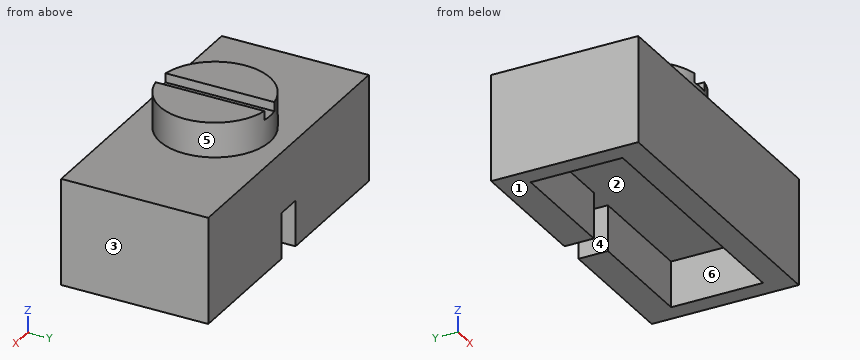
```python
from build123d import *

# Parameters (mm, degrees)
PAD_DEPTH    = 2.5
SKETCH001_W  = 16
SKETCH001_H  = 8
PAD001_DEPTH = 3.3
SKETCH002_R  = 3
PAD002_DEPTH = 5.2
SKETCH003_W  = 1
SKETCH003_H  = 8
POCKET_DEPTH = 0.5


with BuildPart() as part:
    # Sketch → Pad (new body)
    with BuildSketch(Plane.XY):
        Polygon((-8, 4), (-8, -4), (8, -4), (8, 4), (0.7, 4), (0.7, 2.4), (7, 2.4), (7, -2.6), (-7, -2.6), (-7, 2.4), (-0.7, 2.4), (-0.7, 4), align=None)
    extrude(amount=-PAD_DEPTH)

    # Sketch001 → Pad001 (join)
    with BuildSketch(Plane.XY):
        Rectangle(SKETCH001_W, SKETCH001_H)
    extrude(amount=PAD001_DEPTH)

    # Sketch002 → Pad002 (join)
    with BuildSketch(Plane.XY):
        Circle(SKETCH002_R)
    extrude(amount=PAD002_DEPTH)

    # Sketch003 (on Face10 of Pad002) → Pocket (cut)
    with BuildSketch(Plane.XY.offset(5.2)):
        Rectangle(SKETCH003_W, SKETCH003_H)
    extrude(amount=-POCKET_DEPTH, mode=Mode.SUBTRACT)


solid = part.part
```
CAD build for the part. Positions are in the model's coordinates, mm. Face numbers are marked on the shaded views. A direction names the side the tool comes from. Give positions to 0.01 mm unless a question says otherwise; leave off trailing zeros. Write each loop counter-clockwise with the first axis right and the second up, starting at its lowest first coordinate (ties: lowest second). Pieces come first, ordered by that corner, then holes. Notation, with made-up numbers: M 42,6.5 L 65,6.5 A30 cw 65,35.5 Z; hole C 13,-39 d5. An arc over 180 degrees is marked long. Return JSON: item names as keys, results as strings. Group by question number.
(1) Band-saw the part on D-D (x = 5). Give the cut face in (y, z).
(2) 3-axis set-ups, long thin cutter, end or side, ignore diameter. For the marked faces 4, 5 and 6: which of +Z, -Z, +X, -X, +Y, -Y reach the whole face in a straight line?
(3) Band-saw the part on C-C (z = -1). Give the cut face in (x, y).
(4) Flat gauge pins, fed straight in: pin 1 Ø2 at (x, y) = (-5.5, -3) entering from +Z; pin 2 Ø2 at (x, y) = (-0.5, 0.5) entering from -Z; pin 3 Ø0.5 at (x, y) = (0, 0.5) entering from +Z. Where does each tip first touch, or does it go through?
(5) Mould opens along X. For the marked faces 1, 2 and 3 say: pulls with the +X half, pulls with the -X half, needs draft (parallel to the pull), parting line crosses it, or undercut.
(6) Band-saw the part on A-A (x = 0). Give the cut face in (y, z).
(7) Band-saw the part on B-B (y = 0). Give the cut face in (x, z), and give its area (3 significant figures).
(8) Drill centre lines: L1, parallel to Y at x = 3.5, z = -0.25; L2, parallel to X at y = 0.5, z = 4.5; L3, parallel to Z at x = 4.5, y = -3.25. Where is each one in solid material? Low to high. Write a range as [from, to].
Entries:
{
 "1": {"outline": "M -4,-2.5 L -2.6,-2.5 L -2.6,0 L 2.4,0 L 2.4,-2.5 L 4,-2.5 L 4,3.3 L -4,3.3 Z"},
 "2": {"face 4": "-Z, +Y", "face 5": "+Z", "face 6": "-Z"},
 "3": {"outline": "M -8,-4 L 8,-4 L 8,4 L 0.7,4 L 0.7,2.4 L 7,2.4 L 7,-2.6 L -7,-2.6 L -7,2.4 L -0.7,2.4 L -0.7,4 L -8,4 Z"},
 "4": {"pin 1": "stops at z = 3.3", "pin 2": "stops at z = 0", "pin 3": "stops at z = 4.7"},
 "5": {"face 1": "needs draft", "face 2": "undercut", "face 3": "pulls with the +X half"},
 "6": {"outline": "M -4,-2.5 L -2.6,-2.5 L -2.6,0 L 4,0 L 4,3.3 L 3,3.3 L 3,4.7 L -3,4.7 L -3,3.3 L -4,3.3 Z"},
 "7": {"outline": "M -8,-2.5 L -7,-2.5 L -7,0 L 7,0 L 7,-2.5 L 8,-2.5 L 8,3.3 L 3,3.3 L 3,5.2 L 0.5,5.2 L 0.5,4.7 L -0.5,4.7 L -0.5,5.2 L -3,5.2 L -3,3.3 L -8,3.3 Z", "area": "68.7 mm^2"},
 "8": {"L1": "y = [-4, -2.6], [2.4, 4]", "L2": "x = [-2.96, 2.96]", "L3": "z = [-2.5, 3.3]"}
}
